Autodesk Inventor part; units mm, degrees
ref_plane "YZ Plane" through (0, 0, 0) normal (1, 0, 0) x (0, 1, 0)
ref_plane "XZ Plane" through (0, 0, 0) normal (0, 1, 0) x (-1, 0, 0)
ref_plane "XY Plane" through (0, 0, 0) normal (0, 0, 1) x (1, 0, 0)
sketch "Sketch1" plane through (0, 0, 0) normal (0, 0, 1) x (1, 0, 0)
  line L0 (-100.1, -129.95) -> (100.1, -129.95)
  line L1 (100.1, -129.95) -> (100.1, 129.95)
  line L2 (100.1, 129.95) -> (-100.1, 129.95)
  line L3 (-100.1, 129.95) -> (-100.1, -129.95)
  line L4 (-100.1, -129.95) -> (100.1, 129.95) construction
  line L5 (100.1, -129.95) -> (-100.1, 129.95) construction
  point P0 (0, 0)
  dimension "d0" = 200.2
  dimension "d1" = 259.9
extrude "Plate1" add sketch "Sketch1" along normal blind 3.15
sketch "Sketch2" plane through (96.95, -129.95, 3.15) normal (1, 0, 0) x (0, 1, 0)
  line L0 (259.9, 0) -> (0, 0)
  line L1 (0, 0) -> (0, -71)
  line L2 (0, -71) -> (259.9, -71)
  line L3 (259.9, -71) -> (259.9, 0)
edge flange "Flange1" height 71 angle 90 thickness 3.15 bend radius 3.15 thickness toward (1, 0, 0) relief tear relief width 3.15 relief depth 1.575 corner gap 3.15 corner form 0 edges at (100.1, 0, 0) (-100.1, 0, 0) wall of the first edge with corners at (96.95, 129.95, 3.15) (96.95, -129.95, 3.15) (96.95, -129.95, -67.85) (96.95, 129.95, -67.85)
bend "Bend1"
corner "Corner1"
equation "\"d0\" = shield_x"
equation "\"d1\" = shield_z"
equation "\"Thickness\" = shield_t"
equation "\"d3\" = BendReliefWidth"
equation "\"d4\" = BendReliefDepth"
equation "\"d5\" = MinimumRemnant"
equation "\"d6\" = BendRadius"
equation "\"d7\" = shield_y"
equation "\"d9\" = BendRadius"
equation "\"d10\" = CornerReliefSize"
equation "\"d11\" = GapSize"
equation "\"d12\" = JacobiRadiusSize"
equation "\"BendRadius\" = Thickness"
equation "\"BendReliefWidth\" = Thickness"
equation "\"BendReliefDepth\" = 0.5 * Thickness"
equation "\"CornerReliefSize\" = 4 * Thickness"
equation "\"MinimumRemnant\" = 2 * Thickness"
equation "\"TransitionRadius\" = BendRadius"
equation "\"JacobiRadiusSize\" = BendRadius"
equation "\"GapSize\" = Thickness"
equation "\"laserresin\" = 5"
equation "\"st1_thickness\" = 0.91186"
equation "\"st2_thickness\" = 1.5875"
equation "\"al1_thickness\" = 0.79375"
equation "\"al2_thickness\" = 1.5875"
equation "\"bend_factor\" = 2.26205"
equation "\"st1_bend\" = 2.06267"
equation "\"st2_bend\" = 3.591"
equation "\"st3_bend\" = 113.10236"
equation "\"al1_bend\" = 1.7955"
equation "\"al2_bend\" = 3.591"
equation "\"al3_bend\" = 113.10236"
equation "\"acrylic1_thickness\" = 5.88"
equation "\"acrylic2_thickness\" = 3.15"
equation "\"acrylic3_thickness\" = 3.15"
equation "\"corner_small_r\" = 1"
equation "\"corner_big_r\" = 5"
equation "\"linear_bearing_spacing\" = 208"
equation "\"galvo_y_out_offset\" = 27"
equation "\"galvo_y_in_offset\" = 17.5"
equation "\"laser_diameter\" = 13"
equation "\"nema17_x\" = 43"
equation "\"nema17_shaft\" = 24"
equation "\"lmk8uu_x\" = 25"
equation "\"lmk8uu_shaft\" = 15"
equation "\"lmk8uu_z\" = 24"
equation "\"shf8_y\" = 43"
equation "\"acme_nut_d\" = 19.1"
equation "\"acme_nut_upper_d\" = 12.7"
equation "\"handle_spacing\" = 50.8"
equation "\"handle_d\" = 4.7625"
equation "\"handle_hole_d\" = 2.845"
equation "\"handle_projection\" = 20.6375"
equation "\"switch_spacing\" = 19"
equation "\"laser_body_diameter\" = 12"
equation "\"m3_diameter\" = 3"
equation "\"m3_head\" = 6"
equation "\"m4_diameter\" = 4"
equation "\"m5_diameter\" = 5"
equation "\"m5_head\" = 10.3"
equation "\"rivet1_diameter\" = 3.26"
equation "\"rivet2_diameter\" = 3.26"
equation "\"brass_insert_drill\" = 4"
equation "\"m5_brass_insert_drill\" = 6.7"
equation "\"m3_press_nut_drill\" = 4.5"
equation "\"m5_press_nut_drill\" = 6.5"
equation "\"platform_t\" = 1.5875"
equation "\"platform_z\" = 65"
equation "\"platform_fold_x\" = 15"
equation "\"platform_crane_gap\" = 0.1"
equation "\"platform_gap\" = 0.1"
equation "\"platform_upper_y\" = 46.625"
equation "\"crane_t\" = 1.5875"
equation "\"crane_x\" = 233"
equation "\"crane_gap\" = 0.1"
equation "\"tray_t\" = 5.88"
equation "\"tray_to_platform_oversize\" = 0"
equation "\"reservoir_t\" = 0.91186"
equation "\"reservoir_z\" = 35"
equation "\"reservoir_flap_y\" = 20.91186"
equation "\"frame_front_t\" = 0.91186"
equation "\"frame_front_y\" = 56"
equation "\"frame_front_fold\" = 15"
equation "\"frame_gap\" = 0.1"
equation "\"frame_back_t\" = 0.91186"
equation "\"frame_back_x\" = 277.97628"
equation "\"frame_back_y\" = 53.97628"
equation "\"frame_back_z\" = 497.97628"
equation "\"drawer_t\" = 0.91186"
equation "\"drawer_gap\" = 0.1"
equation "\"drawer_reservoir_overlap_x\" = 24.08814"
equation "\"drawer_x\" = 202.02372"
equation "\"drawer_y\" = 73"
equation "\"drawer_seal_y\" = 101"
equation "\"drawer_window_gap\" = 6"
equation "\"foot_t\" = 0.91186"
equation "\"foot_x\" = 198"
equation "\"foot_y\" = 196"
equation "\"laser_holder_t\" = 0.91186"
equation "\"laser_holder_z\" = 75"
equation "\"laser_offset_x\" = 59"
equation "\"laser_offset_y\" = 8.5"
equation "\"subframe_t\" = 0.79375"
equation "\"subframe_x\" = 66"
equation "\"subframe_y\" = 55"
equation "\"shield_t\" = 3.15"
equation "\"shield_x\" = 200.2"
equation "\"shield_y\" = 71"
equation "\"shield_z\" = 259.9"
equation "\"magnet_t\" = 1.6"
equation "\"magnet_w\" = 12.8"
equation "\"d2\" = BendRadius"
equation "\"sae_4_40_diameter\" = 2.845"
properties part number "shield2a"
The listing builds one solid part. Answer for the finished solid, in the listing's coordinates (mm). A direction names the side the tool comes from. Coordinates: 2 decimals unless noted, no trailing zeros. Write each loop counter-clockwise with the first axis right and the second up, starting at its lowest first coordinate (ties: lowest second). Pieces come first, ordered by that corner, then holes. Notation, with made-up numbers: (-28.75, -6.5) - (29.25, -6.5) arc R16 ccw to (29.25, 4.5) - close; hole circle Ø8 at (45.5, 78). An arc over 180 degrees is marked (long way). Return JSON: item names as keys, results as strings. Group by question number.
Q1. The part is cut by section C-C on x = -8. Write down the section's boundary in (y, z), and give its area (3 significant figures).
Q2. Which of the six approach directions +Z, -Z, +X, -X, +Y, -Y give full straight-line access (tool end or side, diameter ignored) to faces 5 (the cylindrical face through (-98.3, 1.82, 1.26)), 6 (the flat face through (-96.95, 2, -35))?
Q3. For a pull along X with two mould halves and no side action, classify faces 1 (the flat face through (-1, 2, 0)), 2 (the flat face through (-100.1, 2, -36)), 3 (the flat face through (100.1, -2, -36)), 4 (the flat face through (96.95, -2, -35)) as +X half, -X half, draft (parallel to the pull), parting line (faces both ways), or undercut.
Q4. The part is cut by section A-A on z = -57. Write down the section's boundary in (x, y), and give its area (3 significant figures).
Q5. The part is cut by section B-B on y = -87. Write down the section's boundary in (x, z), and give its area (3 significant figures).
Q6. A flat-ended cylindrical pin translates along its axis: pin 1 Ø5 at (x, y) = (65.5, 51) entering from -Z. Find the tip coordinate at first contact, or state that the pin passes through.
Q7. Find the intervals of material crossed by line 1 along X through (y, z) = (-31, -63.5); line 2 along Z through (x, y) = (-34, 112); line 3 along X through (y, z) = (99, -0.5), in increasing order. Write a range as [from, to].
Evaluation:
{
 "1": {"outline": "(-129.95, 0) - (129.95, 0) - (129.95, 3.15) - (-129.95, 3.15) - close", "area": "819 mm2"},
 "2": {"face 5": "+Z, -X, +Y, -Y", "face 6": "-Z, +Y, -Y"},
 "3": {"face 1": "undercut", "face 2": "-X half", "face 3": "+X half", "face 4": "undercut"},
 "4": {"outline": "(-100.1, -129.95) - (-96.95, -129.95) - (-96.95, 129.95) - (-100.1, 129.95) - close; (96.95, -129.95) - (100.1, -129.95) - (100.1, 129.95) - (96.95, 129.95) - close", "area": "1,640 mm2"},
 "5": {"outline": "(-100.1, -67.85) - (-96.95, -67.85) - (-96.95, -3.15) arc R3.15 cw to (-93.8, 0) - (93.8, 0) arc R3.15 cw to (96.95, -3.15) - (96.95, -67.85) - (100.1, -67.85) - (100.1, -3.15) arc R6.3 ccw to (93.8, 3.15) - (-93.8, 3.15) arc R6.3 ccw to (-100.1, -3.15) - close", "area": "1,050 mm2"},
 "6": {"pin 1": "stops at z = 0"},
 "7": {"line 1": "x = [-100.1, -96.95], [96.95, 100.1]", "line 2": "z = [0, 3.15]", "line 3": "x = [-99.52, -95.5], [95.5, 99.52]"}
}
